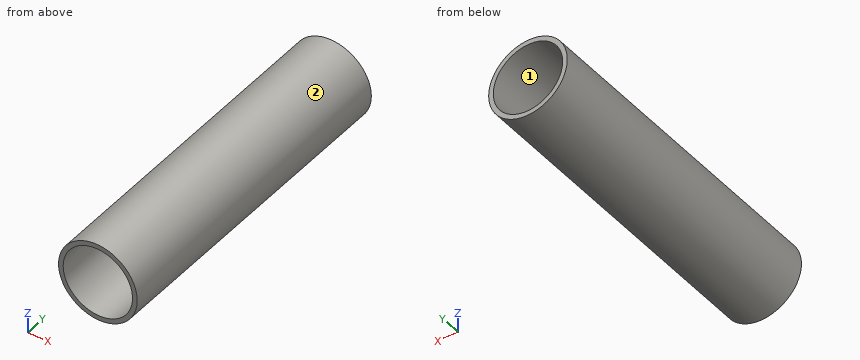
from build123d import *

# Parameters (mm, degrees)
F0_R     = 12.5
F1_DEPTH = 101.6
F2_DEPTH = 25.4
F3_R     = 11.025
F4_DEPTH = 291.084


with BuildPart() as f1:
    # F0 (on Front) → F1 (new body)
    with BuildSketch(Plane.XZ):
        Circle(F0_R)
    extrude(amount=F1_DEPTH)

    # F0 (on Front) → F2 (join)
    with BuildSketch(Plane.XZ):
        Circle(F0_R)
    extrude(amount=F2_DEPTH)

    # F3 (on face) → F4 (cut)
    with BuildSketch(Plane(origin=(0, 0, 0), x_dir=(-1, 0, 0), z_dir=(0, 1, 0))):
        Circle(F3_R)
    extrude(amount=-F4_DEPTH, mode=Mode.SUBTRACT)


solid = f1.part
Verification items for the finished model (mm, model axes). Face numbers are marked on the shaded views. Round coordinates to 2 decimals unless told otherwise and drop trailing zeros. Loops run counter-clockwise (first coordinate to the right, second up) from the corner with the lowest first, then second, coordinate; pieces in that order, holes last. Notation, with made-up numbers: M -6.75,25 L 29.25,25 A32 cw 29.25,53 Z; hole C -19,14 d2. An arc over 180 degrees is marked long. Write each question's results on one line, items separated by ' | '.
1) Mould release check, pull along X, two halves, no side actions. Record for the marked faces 1 and 2: released by +X, released by -X, zero draft, split by the parting line, or undercut.
Checks:
face 1: undercut | face 2: split by the parting line
2) Section check A-A on z = -2.75. Record the boundary of the cut face in (x, y), then the cut area to 3 significant figures.
Checks:
outline: M -12.19,-101.6 L -10.68,-101.6 L -10.68,0 L -12.19,0 Z; M 10.68,-101.6 L 12.19,-101.6 L 12.19,0 L 10.68,0 Z | area: 308 mm2
3) Scan lines: L1, parallel to Z at x = 0, y = -33 (3 decimals); L2, parallel to X at y = -37, z = -0.75; L3, parallel to Z at x = -6.5, y = -67.5. Record each from-to range of solid material in increasing order. Write a range as from..to.
Checks:
L1: z = -12.5..-11.025, 11.025..12.5 | L2: x = -12.48..-11, 11..12.48 | L3: z = -10.68..-8.91, 8.91..10.68
4) Gauge pin test, flat ends, axial feed: P1, Ø3, axis at y = -84.5, z = -9.5, coming from the -X side; P2, Ø2, axis at y = -15, z = -1.5, coming from the +X side; P3, Ø2, axis at y = -40, z = 7, coming from the +X side. Record the tip position at first contact, or that the pin passes through.
Checks:
P1: stops at x = -9.6 | P2: stops at x = 12.49 | P3: stops at x = 10.97
5) Section check C-C on y = -48. Record the boundary of the cut face in (x, z) (3 decimals), then the cut area to 3 significant figures.
Checks:
outline: C 0,0 d25; hole C 0,0 d22.05 | area: 109 mm2
6) Section check B-B on x = 0. Record the boundary of the cut face in (y, z) (3 decimals), then the cut area to 3 significant figures.
Checks:
outline: M -101.6,-12.5 L 0,-12.5 L 0,-11.025 L -101.6,-11.025 Z; M -101.6,11.025 L 0,11.025 L 0,12.5 L -101.6,12.5 Z | area: 300 mm2
